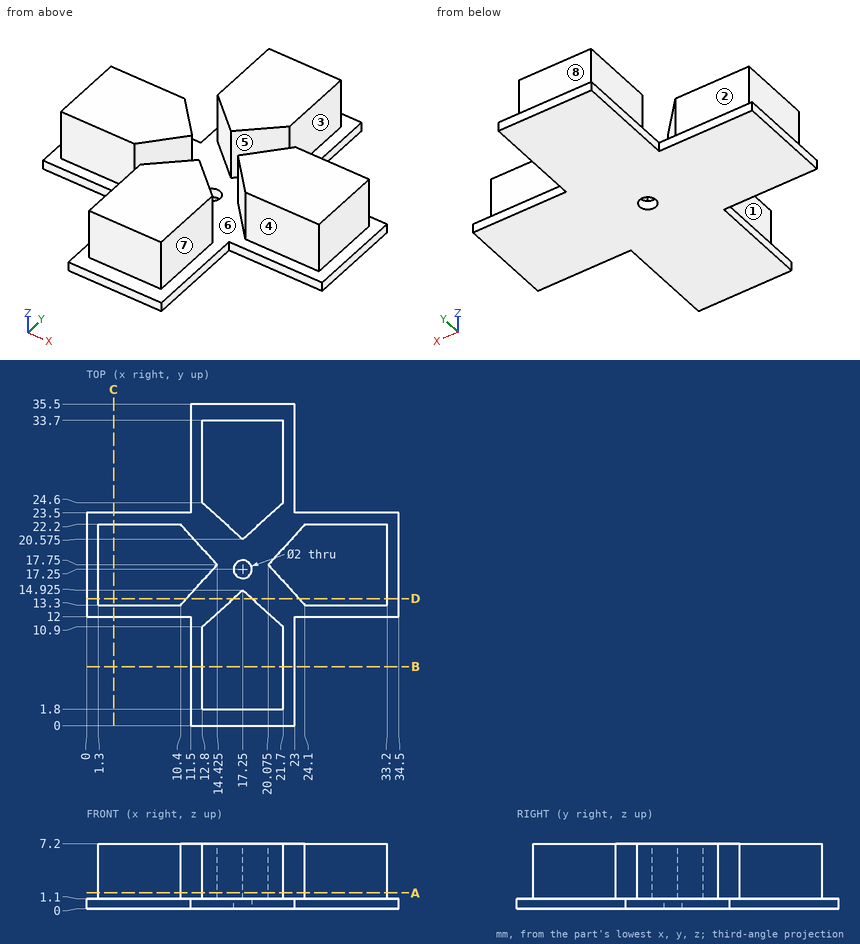
The figure shows three views and two pictorial views of one solid part (mm, origin at its lowest corner). Answer the questions. A direction names the side the tool comes from. Round coordinates to 2 decimals unless told otherwise and drop trailing zeros. Write each loop counter-clockwise with the first axis right and the second up, starting at its lowest first coordinate (ties: lowest second). Pieces come first, ordered by that corner, then holes. Notation, with made-up numbers: (66.25, -26) - (113.25, -26) arc R26 ccw to (113.25, -9) - close; hole circle Ø8 at (69.5, 58). An arc over 180 degrees is marked (long way). Use one line per item in the form item = value. Start each with the question number.
Item 1: A tool of negligible diameter and unlimited length cuts with its end or side. For the marked faces 1, 2, 3, 4 and 5, from which of +Z, -Z, +X, -X, +Y, -Y can it reach the whole face along a straight path? Write none if from no direction.
Item 2: Determine the mould class of the marked faces 6, 7 and 8 for opening direction Y: +Y half, -Y half, draft (parallel to the pull), parting line (faces both ways), or undercut.
Item 3: Find the intervals of material crossed by line 1 (Y direction, x = 17.25, z = 0.3); line 2 (X direction, y = 8, z = 1.5); line 3 (Y direction, x = 27.5, z = 2), in increasing order. Write a range as [from, to].
Item 4: Flat-ended cylindrical pins translate along their axes: pin 1 Ø3 at (y, z) = (6, 4.5) entering from -X; pin 2 Ø3 at (x, z) = (18.5, 4.5) entering from -Y; pin 3 Ø4 at (x, y) = (22, 20) entering from +Z; pin 4 Ø1.2 at (y, z) = (8.5, 0.5) entering from -X. Find the tip coordinate at first contact, or state that the pin passes through.
Item 5: A cutting plane is placed at A-A (z = 1.75). Give the number of separate pieces and of enclosed holes in the cut face.
Item 6: A cutting plane is placed at D-D (y = 14). Write down the section's boundary in (x, z).
Item 7: A cutting plane is placed at B-B (y = 6.5). Write down the section's boundary in (x, z).
Item 8: A cutting plane is placed at C-C (x = 3). Write down the section's boundary in (y, z).
The answers:
q1.face_1 = +Z, -X, -Y
q1.face_2 = +Z, -X, +Y
q1.face_3 = +Z, +X, +Y
q1.face_4 = +Z, +X, -Y
q1.face_5 = +Z
q2.face_6 = undercut
q2.face_7 = draft
q2.face_8 = +Y half
q3.line_1 = [0, 16.25], [18.25, 35.5]
q3.line_2 = [12.8, 21.7]
q3.line_3 = [13.3, 22.2]
q4.pin_1 = 12.8
q4.pin_2 = 1.8
q4.pin_3 = 7.2
q4.pin_4 = 11.5
q5.separate_pieces = 4
q5.enclosed_holes = 0
q6.outline = (0, 0) - (34.5, 0) - (34.5, 1.1) - (33.2, 1.1) - (33.2, 7.2) - (23.47, 7.2) - (23.47, 1.1) - (18.27, 1.1) - (18.27, 7.2) - (16.23, 7.2) - (16.23, 1.1) - (11.03, 1.1) - (11.03, 7.2) - (1.3, 7.2) - (1.3, 1.1) - (0, 1.1) - close
q7.outline = (11.5, 0) - (23, 0) - (23, 1.1) - (21.7, 1.1) - (21.7, 7.2) - (12.8, 7.2) - (12.8, 1.1) - (11.5, 1.1) - close
q8.outline = (12, 0) - (23.5, 0) - (23.5, 1.1) - (22.2, 1.1) - (22.2, 7.2) - (13.3, 7.2) - (13.3, 1.1) - (12, 1.1) - close
